Can you work these out from the model? Positions are in its coordinate system, mm. A direction names the side the tool comes from. Give positions to 0.01 mm unless a question says otherwise; leave off trailing zeros. Loops run counter-clockwise (first coordinate to the right, second up) from the corner with the lowest first, then second, coordinate; pieces in that order, holes last. Notation, with made-up numbers: (38.5, 11.5) - (77.5, 11.5) arc R22 ccw to (77.5, 28.5) - close; hole circle Ø9 at (48, -13). An arc over 180 degrees is marked (long way). Answer in a Markdown table with one row per item.
from build123d import *

# Parameters (mm, degrees)
SKETCH1_R           = 7
BOSS_EXTRUDE1_DEPTH = 25
BOSS_EXTRUDE2_DEPTH = 5
SKETCH1_4_W         = 60
SKETCH1_4_H         = 3
BOSS_EXTRUDE3_DEPTH = 30
SKETCH1_5_W         = 5.181024341
SKETCH1_5_H         = 3
SKETCH1_5_W_2       = 4.652035809
BOSS_EXTRUDE4_DEPTH = 3
SHELL2_START        = 3
SHELL2_OUTLINE_W    = 54
SHELL2_OUTLINE_H    = 35
SHELL2_OUTLINE_R    = 10
SHELL2_DEPTH        = 22
SHELL2_START_2      = -2
SHELL2_2_DEPTH      = 5


# Read off the part's stored shape, not the designer's step: Shell2
with BuildPart() as part:
    # Sketch1 → Boss-Extrude1 (new body)
    # profile 1 of 2: a face of its own
    with BuildSketch(Plane.XY):
        with BuildLine():
            Line((-28.5, 17.5), (14, 17.5))
            Line((14, 17.5), (31.5, 17.5))
            Line((31.5, 17.5), (31.5, -17.5))
            Line((31.5, -17.5), (14, -17.5))
            Line((14, -17.5), (-28.5, -17.5))
            ThreePointArc((-28.5, -17.5), (-11, 0), (-28.5, 17.5))
        make_face()
        with Locations((14, 0)):
            Circle(SKETCH1_R, mode=Mode.SUBTRACT)
    # profile 2 of 2: a face of its own
    with BuildSketch(Plane.XY):
        with BuildLine():
            ThreePointArc((-28.5, 17.5), (-11, 0), (-28.5, -17.5))
            Line((-28.5, -17.5), (-28.5, 17.5))
        make_face()
    extrude(amount=BOSS_EXTRUDE1_DEPTH)

    # Sketch1<3> → Boss-Extrude2 (add)
    with BuildSketch(Plane.XY):
        with BuildLine():
            ThreePointArc((-28.5, 17.5), (-11, 0), (-28.5, -17.5))
            Line((-28.5, -17.5), (-28.5, 17.5))
        make_face()
    extrude(amount=-BOSS_EXTRUDE2_DEPTH)

    # Sketch1<4> → Boss-Extrude3 (add)
    with BuildSketch(Plane.XY):
        with Locations((1.5, 19)):
            Rectangle(SKETCH1_4_W, SKETCH1_4_H)
        with Locations((1.5, -19)):
            Rectangle(SKETCH1_4_W, SKETCH1_4_H)
    extrude(amount=BOSS_EXTRUDE3_DEPTH)

    # Sketch1<5> → Boss-Extrude4 (add)
    with BuildSketch(Plane.XY):
        with Locations((2.590512171, 19)):
            Rectangle(SKETCH1_5_W, SKETCH1_5_H)
        with Locations((2.590512171, -19)):
            Rectangle(SKETCH1_5_W, SKETCH1_5_H)
        with Locations((26.569558343, 19)):
            Rectangle(SKETCH1_5_W_2, SKETCH1_5_H)
        with Locations((26.569558343, -19)):
            Rectangle(SKETCH1_5_W_2, SKETCH1_5_H)
    extrude(amount=-BOSS_EXTRUDE4_DEPTH)

    # Shell2 outline → Shell2 (cut)
    with BuildSketch(Plane.XY.offset(SHELL2_START)):
        with Locations((1.5, 0)):
            Rectangle(SHELL2_OUTLINE_W, SHELL2_OUTLINE_H)
        with Locations((14, 0)):
            Circle(SHELL2_OUTLINE_R, mode=Mode.SUBTRACT)
    extrude(amount=SHELL2_DEPTH, mode=Mode.SUBTRACT)

    # Shell2 2 outline → Shell2 2 (cut)
    with BuildSketch(Plane.XY.offset(SHELL2_START_2)):
        with BuildLine():
            ThreePointArc((-25.5, -14.186260959), (-14, 0), (-25.5, 14.186260959))
            Line((-25.5, 14.186260959), (-25.5, -14.186260959))
        make_face()
    extrude(amount=SHELL2_2_DEPTH, mode=Mode.SUBTRACT)


solid = part.part
Q1. Imagine slicing it at A-A, the plane z = 22. Write out the boundary of the cut face in (x, y), and give its area (3 significant figures).
Checked values:
| item | result |
|---|---|
| outline | (-28.5, -20.5) - (31.5, -20.5) - (31.5, 20.5) - (-28.5, 20.5) - close; circle Ø20 at (14, 0); hole (-25.5, -17.5) - (28.5, -17.5) - (28.5, 17.5) - (-25.5, 17.5) - close; hole circle Ø14 at (14, 0) |
| area | 730 mm² |
Q2. Imagine slicing it at B-B, the plane y = 0. Write out the boundary of the cut face in (x, z), and give its area (3 significant figures).
Checked values:
| item | result |
|---|---|
| outline | (-28.5, -5) - (-11, -5) - (-11, 0) - (7, 0) - (7, 25) - (4, 25) - (4, 3) - (-14, 3) - (-14, -2) - (-25.5, -2) - (-25.5, 25) - (-28.5, 25) - close; (21, 0) - (31.5, 0) - (31.5, 25) - (28.5, 25) - (28.5, 3) - (24, 3) - (24, 25) - (21, 25) - close |
| area | 432 mm² |
Q3. If we mould it in two halves opening along X, with no side actions, what happens to faces 1 (the face through (-22, 0, -5)), 2 (the face through (28.896, -19, -1)), 3 (the face through (1, -17.5, 16))? For each: released by +X, released by -X, zero draft, split by the parting line, or undercut.
Checked values:
| item | result |
|---|---|
| face 1 | zero draft |
| face 2 | released by +X |
| face 3 | undercut |
Q4. If I drill on line 1 (Y direction, x = 14, z = 10); line 2 (Y direction, x = -3.5, z = 22); line 3 (X direction, y = 7.5, z = 19), over which ranges is the centre line in solid material (lowest first)? Write a range as [from, to].
Checked values:
| item | result |
|---|---|
| line 1 | y = [-20.5, -17.5], [-10, -7], [7, 10], [17.5, 20.5] |
| line 2 | y = [-20.5, -17.5], [17.5, 20.5] |
| line 3 | x = [-28.5, -25.5], [7.39, 20.61], [28.5, 31.5] |
Q5. For pin 1 (2.5 mm diameter, centred on x = 25.5, y = -19, fed in from -Z); pin 2 (1.5 mm diameter, centred on y = -19.5, z = -1, fed in from -X); pin 3 (3 mm diameter, centred on x = 18, y = -6.5, fed in from +Z); pin 4 (2.5 mm diameter, centred on y = 19, z = -1, fed in from +X), each with a flat end and sliding along its axis, tell me the tip position at first contact or that it passes through.
Checked values:
| item | result |
|---|---|
| pin 1 | stops at z = -3 |
| pin 2 | stops at x = 0 |
| pin 3 | stops at z = 25 |
| pin 4 | stops at x = 31.5 |
Q6. Imagine slicing it at C-C, the plane x = 14. Write out the boundary of the cut face in (y, z), and give its area (3 significant figures).
Checked values:
| item | result |
|---|---|
| outline | (-20.5, 0) - (-7, 0) - (-7, 25) - (-10, 25) - (-10, 3) - (-17.5, 3) - (-17.5, 30) - (-20.5, 30) - close; (7, 0) - (20.5, 0) - (20.5, 30) - (17.5, 30) - (17.5, 3) - (10, 3) - (10, 25) - (7, 25) - close |
| area | 375 mm² |
Q7. On a 3-axis mill with a long thin cutter (end or side, diameter ignored), from which of +Z, -Z, +X, -X, +Y, -Y can I reach the whole of each face in a straight line? I mean faces 4 (the face through (30, 0, 25)), 5 (the face through (0, 19, -1)), 6 (the face through (28.896, 19, -1)), 7 (the face through (5.181, -19, -1)), 8 (the face through (27, 17.5, -1)). Say none if no direction works.
Checked values:
| item | result |
|---|---|
| face 4 | +Z, +X, -X |
| face 5 | -Z, -X, +Y, -Y |
| face 6 | -Z, +X, +Y, -Y |
| face 7 | -Z, +Y, -Y |
| face 8 | -Z, +X |
Q8. Imagine slicing it at D-D, the plane z = -1. Write out the boundary of the cut face in (x, y).
Checked values:
| item | result |
|---|---|
| outline | (-28.5, -17.5) arc R17.5 ccw to (-28.5, 17.5) - close; (0, -20.5) - (5.18, -20.5) - (5.18, -17.5) - (0, -17.5) - close; (0, 17.5) - (5.18, 17.5) - (5.18, 20.5) - (0, 20.5) - close; (24.24, -20.5) - (28.9, -20.5) - (28.9, -17.5) - (24.24, -17.5) - close; (24.24, 17.5) - (28.9, 17.5) - (28.9, 20.5) - (24.24, 20.5) - close; hole (-25.5, -14.19) arc R14.5 ccw to (-25.5, 14.19) - close |
